Part model, mm, in its own coordinate system. A direction names the side the tool comes from. Give positions to 0.01 mm unless a question says otherwise; leave off trailing zeros. Order: outer loops, then holes, each group sorted by start corner. A loop starts at its lowest first (then second) coordinate and runs counter-clockwise, first axis right, second up. Notation, with made-up numbers: (59, 44.25) - (70, 44.25) arc R20 ccw to (70, 49.25) - close; hole circle Ø3 at (75, -1). An arc over 180 degrees is marked (long way). Use one line per item in the form item = value. Start each with the question number.
1. Band-saw the part on C-C, the plane z = 0.3. State how many separate pieces and enclosed holes the cut face has, plus the area to 3 significant figures.
2. Band-saw the part on D-D, the plane x = 16. List the corners of the cut face in (y, z), plus the area to 3 significant figures.
3. Band-saw the part on A-A, the plane y = -15.5. List the corners of the cut face in (x, z), plus the area to 3 significant figures.
4. Pin check, flat tips, straight feed: P1, Ø0.9, axis at x = 0.08, y = -42.41, coming from the +Z side; P2, Ø1, axis at y = 23, z = 1.5, coming from the +X side. Stop position of each tip, or through.
5. Tool access for faces 4 (the face through (-19.916, -15, 1)), 5 (the face through (0, 18.697, 1)): list every direction of +Z, -Z, +X, -X, +Y, -Y with a clear straight run to the whole face (end or side of a thin tool).
6. Band-saw the part on B-B, the plane x = 7. List the corners of the cut face in (y, z), plus the area to 3 significant figures.
7. Pull direction Y, two halves, no side cores. Call faces 1 (the face through (-1.416, 23, 1)), 2 (the face through (-17.065, 22.828, 1.014)), 3 (the face through (19.083, 12.619, 0.986)): +Y half, -Y half, draft (parallel to the pull), parting line (faces both ways), or undercut.
8. Drill centre lines: line 1 (Y direction, x = 5.5, z = 1.3); line 2 (Y direction, x = -4, z = 0.45); line 3 (Y direction, x = -6, z = 1.65). Where is each one in solid material? Low to high.
from build123d import *

# Parameters (mm, degrees)
CROQUIS1_W              = 40
CROQUIS1_H              = 70
SALIENTE_EXTRUIR1_DEPTH = 2
REDONDEO1_R             = 10
CORTAR_EXTRUIR1_REACH   = 50.558
CROQUIS2_R              = 0.75
CORTAR_EXTRUIR2_REACH   = 50.558
CROQUIS3_W              = 7
CROQUIS3_H              = 2
CORTAR_EXTRUIR3_REACH   = 50.558
CROQUIS4_W              = 3
CROQUIS4_H              = 5.138146931
CROQUIS4_W_2            = 7
CROQUIS4_H_2            = 9
CROQUIS4_W_3            = 9
CROQUIS4_H_3            = 4


with BuildPart() as part:
    # Croquis1 → Saliente-Extruir1 (new body)
    with BuildSketch(Plane.XY):
        with Locations((0.083817915, -9.164456233)):
            Rectangle(CROQUIS1_W, CROQUIS1_H)
    extrude(amount=SALIENTE_EXTRUIR1_DEPTH)

    # Redondeo1
    redondeo1_edges = [part.edges().sort_by_distance(p)[0] for p in [
        (-19.916182085, 25.835543767, 1),
        (20.083817915, 25.835543767, 1),
    ]]
    fillet(redondeo1_edges, radius=REDONDEO1_R)

    # Croquis2 → Cortar-Extruir1 (cut, up to next)
    with BuildSketch(Plane(origin=(0, 0, 0), x_dir=(-1, 0, 0), z_dir=(0, 0, -1)), mode=Mode.PRIVATE) as cortar_extruir1_sk1:
        with Locations((-5.583817915, 24.085543767)):
            Circle(CROQUIS2_R)
    cortar_extruir1_tool1 = extrude(cortar_extruir1_sk1.sketch, amount=-CORTAR_EXTRUIR1_REACH, mode=Mode.PRIVATE) & part.part
    # Croquis2 → Cortar-Extruir1 (cut, up to next)
    with BuildSketch(Plane(origin=(0, 0, 0), x_dir=(-1, 0, 0), z_dir=(0, 0, -1)), mode=Mode.PRIVATE) as cortar_extruir1_sk2:
        with Locations((5.416182085, 24.085543767)):
            Circle(CROQUIS2_R)
    cortar_extruir1_tool2 = extrude(cortar_extruir1_sk2.sketch, amount=-CORTAR_EXTRUIR1_REACH, mode=Mode.PRIVATE) & part.part
    # Croquis2 → Cortar-Extruir1 (cut, up to next)
    with BuildSketch(Plane(origin=(0, 0, 0), x_dir=(-1, 0, 0), z_dir=(0, 0, -1)), mode=Mode.PRIVATE) as cortar_extruir1_sk3:
        with Locations((-18.183817915, -42.414456233)):
            Circle(CROQUIS2_R)
    cortar_extruir1_tool3 = extrude(cortar_extruir1_sk3.sketch, amount=-CORTAR_EXTRUIR1_REACH, mode=Mode.PRIVATE) & part.part
    # Croquis2 → Cortar-Extruir1 (cut, up to next)
    with BuildSketch(Plane(origin=(0, 0, 0), x_dir=(-1, 0, 0), z_dir=(0, 0, -1)), mode=Mode.PRIVATE) as cortar_extruir1_sk4:
        with Locations((-0.083817915, -42.414456233)):
            Circle(CROQUIS2_R)
    cortar_extruir1_tool4 = extrude(cortar_extruir1_sk4.sketch, amount=-CORTAR_EXTRUIR1_REACH, mode=Mode.PRIVATE) & part.part
    # Croquis2 → Cortar-Extruir1 (cut, up to next)
    with BuildSketch(Plane(origin=(0, 0, 0), x_dir=(-1, 0, 0), z_dir=(0, 0, -1)), mode=Mode.PRIVATE) as cortar_extruir1_sk5:
        with Locations((18.016182085, -42.414456233)):
            Circle(CROQUIS2_R)
    cortar_extruir1_tool5 = extrude(cortar_extruir1_sk5.sketch, amount=-CORTAR_EXTRUIR1_REACH, mode=Mode.PRIVATE) & part.part
    # Croquis2 → Cortar-Extruir1 (cut, up to next)
    with BuildSketch(Plane(origin=(0, 0, 0), x_dir=(-1, 0, 0), z_dir=(0, 0, -1)), mode=Mode.PRIVATE) as cortar_extruir1_sk6:
        with Locations((-18.333817915, 12.585543767)):
            Circle(CROQUIS2_R)
    cortar_extruir1_tool6 = extrude(cortar_extruir1_sk6.sketch, amount=-CORTAR_EXTRUIR1_REACH, mode=Mode.PRIVATE) & part.part
    # Croquis2 → Cortar-Extruir1 (cut, up to next)
    with BuildSketch(Plane(origin=(0, 0, 0), x_dir=(-1, 0, 0), z_dir=(0, 0, -1)), mode=Mode.PRIVATE) as cortar_extruir1_sk7:
        with Locations((-18.333817915, -22.414456233)):
            Circle(CROQUIS2_R)
    cortar_extruir1_tool7 = extrude(cortar_extruir1_sk7.sketch, amount=-CORTAR_EXTRUIR1_REACH, mode=Mode.PRIVATE) & part.part
    # Croquis2 → Cortar-Extruir1 (cut, up to next)
    with BuildSketch(Plane(origin=(0, 0, 0), x_dir=(-1, 0, 0), z_dir=(0, 0, -1)), mode=Mode.PRIVATE) as cortar_extruir1_sk8:
        with Locations((18.166182085, 12.585543767)):
            Circle(CROQUIS2_R)
    cortar_extruir1_tool8 = extrude(cortar_extruir1_sk8.sketch, amount=-CORTAR_EXTRUIR1_REACH, mode=Mode.PRIVATE) & part.part
    # Croquis2 → Cortar-Extruir1 (cut, up to next)
    with BuildSketch(Plane(origin=(0, 0, 0), x_dir=(-1, 0, 0), z_dir=(0, 0, -1)), mode=Mode.PRIVATE) as cortar_extruir1_sk9:
        with Locations((18.166182085, -22.414456233)):
            Circle(CROQUIS2_R)
    cortar_extruir1_tool9 = extrude(cortar_extruir1_sk9.sketch, amount=-CORTAR_EXTRUIR1_REACH, mode=Mode.PRIVATE) & part.part
    add(cortar_extruir1_tool1.solids().sort_by_distance((5.583818, 24.085544, 0))[0], mode=Mode.SUBTRACT)
    add(cortar_extruir1_tool2.solids().sort_by_distance((-5.416182, 24.085544, 0))[0], mode=Mode.SUBTRACT)
    add(cortar_extruir1_tool3.solids().sort_by_distance((18.183818, -42.414456, 0))[0], mode=Mode.SUBTRACT)
    add(cortar_extruir1_tool4.solids().sort_by_distance((0.083818, -42.414456, 0))[0], mode=Mode.SUBTRACT)
    add(cortar_extruir1_tool5.solids().sort_by_distance((-18.016182, -42.414456, 0))[0], mode=Mode.SUBTRACT)
    add(cortar_extruir1_tool6.solids().sort_by_distance((18.333818, 12.585544, 0))[0], mode=Mode.SUBTRACT)
    add(cortar_extruir1_tool7.solids().sort_by_distance((18.333818, -22.414456, 0))[0], mode=Mode.SUBTRACT)
    add(cortar_extruir1_tool8.solids().sort_by_distance((-18.166182, 12.585544, 0))[0], mode=Mode.SUBTRACT)
    add(cortar_extruir1_tool9.solids().sort_by_distance((-18.166182, -22.414456, 0))[0], mode=Mode.SUBTRACT)

    # Croquis3 → Cortar-Extruir2 (cut, up to next)
    with BuildSketch(Plane(origin=(0, 0, 0), x_dir=(-1, 0, 0), z_dir=(0, 0, -1)), mode=Mode.PRIVATE) as cortar_extruir2_sk1:
        with Locations((-0.083817915, 19.697396836)):
            Rectangle(CROQUIS3_W, CROQUIS3_H)
    cortar_extruir2_tool1 = extrude(cortar_extruir2_sk1.sketch, amount=-CORTAR_EXTRUIR2_REACH, mode=Mode.PRIVATE) & part.part
    add(cortar_extruir2_tool1.solids().sort_by_distance((0.083818, 19.697397, 0))[0], mode=Mode.SUBTRACT)

    # Croquis4 → Cortar-Extruir3 (cut, up to next)
    with BuildSketch(Plane(origin=(0, 0, 0), x_dir=(-1, 0, 0), z_dir=(0, 0, -1)), mode=Mode.PRIVATE) as cortar_extruir3_sk1:
        with Locations((-0.083817915, 23.266470302)):
            Rectangle(CROQUIS4_W, CROQUIS4_H)
    cortar_extruir3_tool1 = extrude(cortar_extruir3_sk1.sketch, amount=-CORTAR_EXTRUIR3_REACH, mode=Mode.PRIVATE) & part.part
    # Croquis4 → Cortar-Extruir3 (cut, up to next)
    with BuildSketch(Plane(origin=(0, 0, 0), x_dir=(-1, 0, 0), z_dir=(0, 0, -1)), mode=Mode.PRIVATE) as cortar_extruir3_sk2:
        with Locations((-9.583817915, -14.664456233)):
            Rectangle(CROQUIS4_W_2, CROQUIS4_H_2)
    cortar_extruir3_tool2 = extrude(cortar_extruir3_sk2.sketch, amount=-CORTAR_EXTRUIR3_REACH, mode=Mode.PRIVATE) & part.part
    # Croquis4 → Cortar-Extruir3 (cut, up to next)
    with BuildSketch(Plane(origin=(0, 0, 0), x_dir=(-1, 0, 0), z_dir=(0, 0, -1)), mode=Mode.PRIVATE) as cortar_extruir3_sk3:
        with Locations((3.416182085, -24.664456233)):
            Rectangle(CROQUIS4_W_3, CROQUIS4_H_3)
    cortar_extruir3_tool3 = extrude(cortar_extruir3_sk3.sketch, amount=-CORTAR_EXTRUIR3_REACH, mode=Mode.PRIVATE) & part.part
    add(cortar_extruir3_tool1.solids().sort_by_distance((0.083818, 23.26647, 0))[0], mode=Mode.SUBTRACT)
    add(cortar_extruir3_tool2.solids().sort_by_distance((9.583818, -14.664456, 0))[0], mode=Mode.SUBTRACT)
    add(cortar_extruir3_tool3.solids().sort_by_distance((-3.416182, -24.664456, 0))[0], mode=Mode.SUBTRACT)


solid = part.part
From the geometry:
q1.separate_pieces = 1
q1.enclosed_holes = 11
q1.area = 2,610 mm²
q2.outline = (-44.16, 0) - (23.9, 0) - (23.9, 2) - (-44.16, 2) - close
q2.area = 136 mm²
q3.outline = (-19.92, 0) - (6.08, 0) - (6.08, 2) - (-19.92, 2) - close; (13.08, 0) - (20.08, 0) - (20.08, 2) - (13.08, 2) - close
q3.area = 66.0 mm²
q4.P1 = through
q4.P2 = 17.54
q5.face_4 = +Z, -Z, -X, +Y, -Y
q5.face_5 = +Z, -Z
q6.outline = (-44.16, 0) - (-19.16, 0) - (-19.16, 2) - (-44.16, 2) - close; (-10.16, 0) - (25.84, 0) - (25.84, 2) - (-10.16, 2) - close
q6.area = 122 mm²
q7.face_1 = draft
q7.face_2 = +Y half
q7.face_3 = undercut
q8.line_1 = -44.16 to 23.34, 24.83 to 25.84
q8.line_2 = -44.16 to -26.66, -22.66 to 25.84
q8.line_3 = -44.16 to -26.66, -22.66 to 23.61, 24.56 to 25.84
